```python
from build123d import *


with BuildPart() as part:
    # Skizze1 → Rotation1 (revolve)
    with BuildSketch(Plane(origin=(0, 0, 0), x_dir=(1, 0, 0), z_dir=(0, 1, 0)), mode=Mode.PRIVATE) as rotation1_sk:
        Polygon((0, 20), (8, 20), (8, 0), (16, 0), (16, -123.535), (30.4, -123.535), (30.4, -145.535), (0, -145.535), align=None)
    revolve(rotation1_sk.sketch.rotate(Axis((0, 0, -20), (0, 0, 1)), 180), axis=Axis((0, 0, -20), (0, 0, 1)))  # turned: the seam where the file's is


solid = part.part
```
Work out the finished part from the listing and answer in its coordinate system (mm). A direction names the side the tool comes from. Round coordinates to 2 decimals unless told otherwise and drop trailing zeros. Loops run counter-clockwise (first coordinate to the right, second up) from the corner with the lowest first, then second, coordinate; pieces in that order, holes last. Notation, with made-up numbers: M -34.75,-33 L 9.25,-33 A30 ccw 9.25,-5 Z; hole C 31,-3 d9. An arc over 180 degrees is marked long. One line per question, with ' | ' between items.
Q1. Find section C-C, the plane z = 106. Give the vertices of the cut face in (x, y), then the cut area to 3 significant figures.
Conclusion:
outline: C 0,0 d32 | area: 804 mm2
Q2. Consider line 1 along Z through (x, y) = (16.5, 24) (3 decimals); line 2 along Z through (x, y) = (-11, 10.5) (3 decimals); line 3 along X through (y, z) = (1, 28). Determine where each line is inside the solid, lowest interval first. Write a range as from..to.
Conclusion:
line 1: z = 123.535..145.535 | line 2: z = 0..145.535 | line 3: x = -15.97..15.97
Q3. A tool of negligible diameter and unlimited length cuts with its end or side. For faces 1 (the cylindrical face through (1.73, 7.81, -9.86)), 2 (the flat face through (0, 0, 145.535)), from which of +Z, -Z, +X, -X, +Y, -Y can it reach the whole face along a straight path? Write none if from no direction.
Conclusion:
face 1: -Z | face 2: +Z, +X, -X, +Y, -Y
Q4. Find section A-A, the plane y = 0. Give the vertices of the cut face in (x, z) (3 decimals).
Conclusion:
outline: M -30.4,123.535 L -16,123.535 L -16,0 L -8,0 L -8,-20 L 8,-20 L 8,0 L 16,0 L 16,123.535 L 30.4,123.535 L 30.4,145.535 L -30.4,145.535 Z
Q5. Each of these flat-tipped pins is pushed along its axis until it touches: pin 1 Ø12 at (y, z) = (17, -0.5) entering from -X; pin 2 Ø4 at (x, z) = (-8, 125) entering from -Y; pin 3 Ø1.5 at (y, z) = (15, 41) entering from -X. Where does it stop, or does it pass through?
Conclusion:
pin 1: stops at x = -11.6 | pin 2: stops at y = -29.8 | pin 3: stops at x = -7.28
Q6. Find section D-D, the plane x = -14.5. Give the vertices of the cut face in (y, z) (3 decimals).
Conclusion:
outline: M -26.719,123.535 L -6.764,123.535 L -6.764,0 L 6.764,0 L 6.764,123.535 L 26.719,123.535 L 26.719,145.535 L -26.719,145.535 Z
